```python
from build123d import *

# Parameters (mm, degrees)
BOSS_EXTRUDE1_DEPTH = 3
SKETCH4_R           = 6.5
CUT_EXTRUDE1_DEPTH  = 3
SKETCH5_R           = 3
SKETCH5_R_2         = 1.5
CUT_EXTRUDE2_DEPTH  = 3
SKETCH6_W           = 3
SKETCH6_H           = 7
CUT_EXTRUDE3_DEPTH  = 3
SKETCH7_W           = 3
SKETCH7_H           = 5
CUT_EXTRUDE4_DEPTH  = 3


with BuildPart() as part:
    # Sketch2 → Boss-Extrude1 (new body)
    with BuildSketch(Plane(origin=(0, 0, 0), x_dir=(1, 0, 0), z_dir=(0, 1, 0))):
        with BuildLine():
            Line((-3.583885407, 15.877073113), (62.416114593, 15.877073113))
            ThreePointArc((62.416114593, 15.877073113), (63.830328155, 15.291286675), (64.416114593, 13.877073113))
            Line((64.416114593, 13.877073113), (64.416114593, -0.122926887))
            ThreePointArc((64.416114593, -0.122926887), (63.830328155, -1.53714045), (62.416114593, -2.122926887))
            Line((62.416114593, -2.122926887), (-3.583885407, -2.122926887))
            ThreePointArc((-3.583885407, -2.122926887), (-4.99809897, -1.53714045), (-5.583885407, -0.122926887))
            Line((-5.583885407, -0.122926887), (-5.583885407, 13.877073113))
            ThreePointArc((-5.583885407, 13.877073113), (-4.99809897, 15.291286675), (-3.583885407, 15.877073113))
        make_face()
    extrude(amount=BOSS_EXTRUDE1_DEPTH)

    # Sketch4 → Cut-Extrude1 (cut)
    with BuildSketch(Plane(origin=(0, 3, 0), x_dir=(1, 0, 0), z_dir=(0, 1, 0))):
        with Locations(Location((15.816114593, 6.877073113, 0), (0, 0, 270))):
            Circle(SKETCH4_R)
    extrude(amount=-CUT_EXTRUDE1_DEPTH, mode=Mode.SUBTRACT)

    # Sketch5 → Cut-Extrude2 (cut)
    with BuildSketch(Plane(origin=(0, 3, 0), x_dir=(1, 0, 0), z_dir=(0, 1, 0))):
        with Locations((21.296114593, 6.977073113)):
            Circle(SKETCH5_R)
        with Locations(Location((42.816114593, 6.977073113, 0), (0, 0, 270))):
            Circle(SKETCH5_R_2)
    extrude(amount=-CUT_EXTRUDE2_DEPTH, mode=Mode.SUBTRACT)

    # Sketch6 → Cut-Extrude3 (cut)
    with BuildSketch(Plane(origin=(0, 3, 0), x_dir=(1, 0, 0), z_dir=(0, 1, 0))):
        with Locations((1.416114593, 12.377073113)):
            Rectangle(SKETCH6_W, SKETCH6_H)
        with Locations((57.416114593, 12.377073113)):
            Rectangle(SKETCH6_W, SKETCH6_H)
    extrude(amount=-CUT_EXTRUDE3_DEPTH, mode=Mode.SUBTRACT)

    # Sketch7 → Cut-Extrude4 (cut)
    with BuildSketch(Plane(origin=(0, 3, 0), x_dir=(1, 0, 0), z_dir=(0, 1, 0))):
        with Locations((60.416114593, 0.377073113)):
            Rectangle(SKETCH7_W, SKETCH7_H)
        with Locations((-1.583885407, 0.377073113)):
            Rectangle(SKETCH7_W, SKETCH7_H)
    extrude(amount=-CUT_EXTRUDE4_DEPTH, mode=Mode.SUBTRACT)


solid = part.part
```
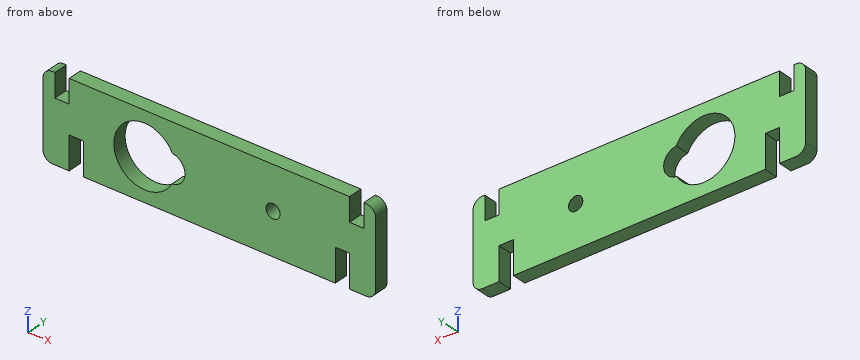
Input: part model. Units: mm. Frame: model coordinates. Coordinates: 2 decimals unless noted, no trailing zeros. Write each loop counter-clockwise with the first axis right and the second up, starting at its lowest first coordinate (ties: lowest second). Pieces come first, ordered by that corner, then holes.
1) Pin query (flat end, axial travel): pin 1 Ø0.9 at (x, y) = (0.5, 1.5) entering from -Z. Return the tip coordinate at first contact, or that it passes through.
2) Section A-A on z = -6.5. Output: boundary loops of the cut face in (x, y), and give its area (3 significant figures).
3) Section B-B on x = 10. Output: boundary loops of the cut face in (y, z), and give its area (3 significant figures).
4) Material intervals for line 1 along X through (y, z) = (0.25, -0.25); line 2 along X through (y, z) = (1.7, -14); line 3 along X through (y, z) = (1.45, -1.25), sorted ascending.
5) Section C-C on y = 1.1. Output: boundary loops of the cut face in (x, z), and give its area (3 significant figures).
6) Section D-D on x = 58. Output: boundary loops of the cut face in (y, z), and give its area (3 significant figures).
Check result:
1. pin 1: stops at z = -8.88
2. outline: (-5.58, 0) - (9.33, 0) - (9.33, 3) - (-5.58, 3) - close; (24.26, 0) - (41.39, 0) - (41.39, 3) - (24.26, 3) - close; (44.24, 0) - (64.42, 0) - (64.42, 3) - (44.24, 3) - close
2. area: 157 mm2
3. outline: (0, -15.88) - (3, -15.88) - (3, -9.78) - (0, -9.78) - close; (0, -3.97) - (3, -3.97) - (3, 2.12) - (0, 2.12) - close
3. area: 36.6 mm2
4. line 1: x = -5.58 to -3.08, -0.08 to 58.92, 61.92 to 64.42
4. line 2: x = -5.58 to -0.08, 2.92 to 55.92, 58.92 to 64.41
4. line 3: x = -5.58 to -3.08, -0.08 to 12.56, 19.07 to 58.92, 61.92 to 64.42
5. outline: (-5.58, -13.88) arc R2 ccw to (-3.58, -15.88) - (-0.08, -15.88) - (-0.08, -8.88) - (2.92, -8.88) - (2.92, -15.88) - (55.92, -15.88) - (55.92, -8.88) - (58.92, -8.88) - (58.92, -15.88) - (62.42, -15.88) arc R2 ccw to (64.42, -13.88) - (64.42, 0.12) arc R2 ccw to (62.42, 2.12) - (61.92, 2.12) - (61.92, -2.88) - (58.92, -2.88) - (58.92, 2.12) - (-0.08, 2.12) - (-0.08, -2.88) - (-3.08, -2.88) - (-3.08, 2.12) - (-3.58, 2.12) arc R2 ccw to (-5.58, 0.12) - close; hole (21.53, -9.97) arc R3 ccw to (21.64, -4) arc R6.5 ccw (long way) to start; hole circle Ø3 at (42.82, -6.98)
5. area: 1,040 mm2
6. outline: (0, -8.88) - (3, -8.88) - (3, 2.12) - (0, 2.12) - close
6. area: 33.0 mm2
